Here's how the part is built. I have some questions about the finished solid (model axes, mm). Coordinates: 2 decimals unless noted, no trailing zeros. Loops run counter-clockwise (first coordinate to the right, second up) from the corner with the lowest first, then second, coordinate; pieces in that order, holes last. Notation, with made-up numbers: (23.25, 82.5) - (54.25, 82.5) arc R24 ccw to (54.25, 120.5) - close; hole circle Ø5 at (-36.5, 13.5). An arc over 180 degrees is marked (long way). Use a Markdown table: item, result.
```python
from build123d import *

# Parameters (mm, degrees)
SKETCH1_R           = 33.3375
BOSS_EXTRUDE1_DEPTH = 25.4
SKETCH2_R           = 3.556
CUT_EXTRUDE1_DEPTH  = 54.553130744
SKETCH3_R           = 3.175
CUT_EXTRUDE2_DEPTH  = 54.553130744


with BuildPart() as part:
    # Sketch1 → Boss-Extrude1 (new body)
    with BuildSketch(Plane(origin=(0, 0, 0), x_dir=(1, 0, 0), z_dir=(0, 1, 0))):
        with Locations(Location((0, 0, 0), (0, 0, 270))):
            Circle(SKETCH1_R)
    extrude(amount=BOSS_EXTRUDE1_DEPTH)

    # Sketch2 → Cut-Extrude1 (cut, through all)
    with BuildSketch(Plane(origin=(0, 25.4, 0), x_dir=(1, 0, 0), z_dir=(0, 1, 0))):
        with Locations(Location((0, 0, 0), (0, 0, 270))):
            Circle(SKETCH2_R)
    extrude(amount=-CUT_EXTRUDE1_DEPTH, mode=Mode.SUBTRACT)

    # Sketch3 → Cut-Extrude2 (cut, through all)
    with BuildSketch(Plane(origin=(0, 25.4, 0), x_dir=(-1, 0, 0), z_dir=(0, 1, 0))):
        with Locations(Location((13.462, 0, 0), (0, 0, 90))):
            Circle(SKETCH3_R)
        with Locations(Location((-13.462, 0, 0), (0, 0, 270))):
            Circle(SKETCH3_R)
    extrude(amount=-CUT_EXTRUDE2_DEPTH, mode=Mode.SUBTRACT)


solid = part.part
```
Q1. I want a section at A-A, the plane z = 0. Write out the boundary of the cut face in (x, y), then the cut area to 3 significant figures.
Check values:
| item | result |
|---|---|
| outline | (-33.34, 0) - (-16.64, 0) - (-16.64, 25.4) - (-33.34, 25.4) - close; (-10.29, 0) - (-3.56, 0) - (-3.56, 25.4) - (-10.29, 25.4) - close; (3.56, 0) - (10.29, 0) - (10.29, 25.4) - (3.56, 25.4) - close; (16.64, 0) - (33.34, 0) - (33.34, 25.4) - (16.64, 25.4) - close |
| area | 1,190 mm^2 |
Q2. Please list where these lines run through material, in increasing order: L1, parallel to X at y = 17.5, z = 0; L2, parallel to X at y = 11.25, z = 2.5; L3, parallel to Z at x = 15, y = 19.25. Write a range as from..to.
Check values:
| item | result |
|---|---|
| L1 | -33.34..-16.64, -10.29..-3.56, 3.56..10.29, 16.64..33.34 |
| L2 | -33.24..-15.42, -11.5..-2.53, 2.53..11.5, 15.42..33.24 |
| L3 | -29.77..-2.78, 2.78..29.77 |
Q3. I want a section at B-B, the plane x = 0. Write out the boundary of the cut face in (y, z).
Check values:
| item | result |
|---|---|
| outline | (0, -33.34) - (25.4, -33.34) - (25.4, -3.56) - (0, -3.56) - close; (0, 3.56) - (25.4, 3.56) - (25.4, 33.34) - (0, 33.34) - close |
Q4. I want a section at D-D, the plane x = 8. Write out the boundary of the cut face in (y, z), then the cut area to 3 significant figures.
Check values:
| item | result |
|---|---|
| outline | (0, -32.36) - (25.4, -32.36) - (25.4, 32.36) - (0, 32.36) - close |
| area | 1,640 mm^2 |
Q5. I want a section at C-C, the plane y = 2.5. Give the number of separate pieces and of enclosed holes in the cut face, then the cut area to 3 significant figures.
Check values:
| item | result |
|---|---|
| separate pieces | 1 |
| enclosed holes | 3 |
| area | 3,390 mm^2 |
Q6. If we mould it in two halves opening along X, with no side actions, what happens to faces 1 (the face through (-16.56, 12.88, -0.69)), 2 (the face through (-7, 25.4, 0)), 3 (the face through (10.01, 12.52, 31.8))? For each: pulls with the +X half, pulls with the -X half, needs draft (parallel to the pull), parting line crosses it, or undercut.
Check values:
| item | result |
|---|---|
| face 1 | undercut |
| face 2 | needs draft |
| face 3 | parting line crosses it |
Q7. Will these pins go through, and if not, where does the flat tip stop? P1, Ø3, axis at x = 13, y = 6.5, coming from the +Z side; P2, Ø1.5, axis at x = -19.5, z = 10.5, coming from the -Y side; P3, Ø6, axis at y = 3, z = -2, coming from the -X side; P4, Ø1, axis at x = 18.5, y = 4.5, coming from the +Z side.
Check values:
| item | result |
|---|---|
| P1 | z = 31.29 |
| P2 | y = 0 |
| P3 | x = -33.34 |
| P4 | z = 28.06 |
